Read the model definition and answer for the solid it produces. Units are mm, in the model's axes. Coordinates: 2 decimals unless noted, no trailing zeros. Write each loop counter-clockwise with the first axis right and the second up, starting at its lowest first coordinate (ties: lowest second). Pieces come first, ordered by that corner, then holes.
(1) The part is cut by section B-B, the plane x = 23. Determine the outline of the cut face in (y, z), and give its area (3 significant figures).
(2) The part is cut by section C-C, the plane z = 420. Determine the outline of the cut face in (x, y), and give its area (3 significant figures).
(3) Straight lines are drawn through the part: line 1 along Y through (x, z) = (0, 478.5); line 2 along X through (y, z) = (4, 572.5). For each, find the intervals that lie inside material, in ascending order.
(4) Given pin 1 (1 mm diameter, centred on x = 3, z = 241, fed in from +Y); pin 2 (2 mm diameter, centred on x = -31, y = 34.5, fed in from -Z) (3 decimals); pin 3 (6 mm diameter, centred on y = -1, z = 731, fed in from -X); pin 4 (1 mm diameter, centred on x = 9.5, z = 522.5, fed in from +Y), each flat-ended and moving along its own axis, determine where each tip first touches the part or whether it passes through.
(5) The part is cut by section A-A, the plane y = 31.5. Determine the outline of the cut face in (x, z).
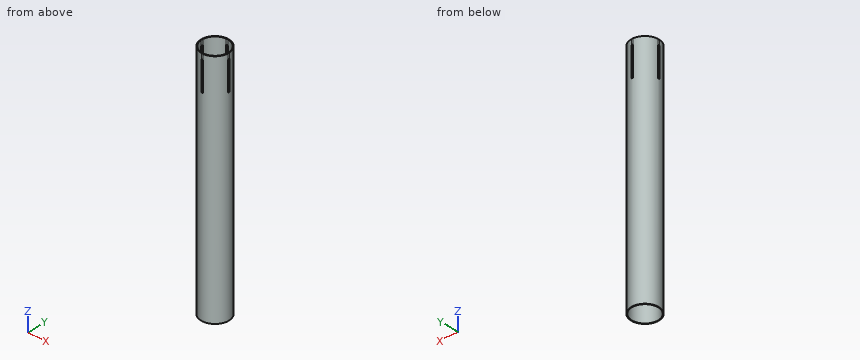
```python
from build123d import *
from build123d.topology import SkipClean

# Parameters (mm, degrees)
SKETCH1_R           = 50.8
SKETCH1_R_2         = 48.26
BOSS_EXTRUDE1_DEPTH = 863.6
CUT_EXTRUDE1_START  = -127
CUT_EXTRUDE1_DEPTH  = 127
BOSS_EXTRUDE2_START = -19.05
BOSS_EXTRUDE2_DEPTH = 19.05


with BuildPart() as part:
    # Sketch1 → Boss-Extrude1 (new body)
    with BuildSketch(Plane.XY):
        Circle(SKETCH1_R)
        Circle(SKETCH1_R_2, mode=Mode.SUBTRACT)
    extrude(amount=BOSS_EXTRUDE1_DEPTH)

    # Sketch2 → Cut-Extrude1 (cut)
    with BuildSketch(Plane.XY.offset(863.6).offset(CUT_EXTRUDE1_START)):
        with BuildLine():
            Line((-3.175, 50.700684167), (-3.175, 48.155445954))
            ThreePointArc((-3.175, 48.155445954), (0, 48.26), (3.175, 48.155445954))
            Line((3.175, 48.155445954), (3.175, 50.700684167))
            ThreePointArc((3.175, 50.700684167), (0, 50.8), (-3.175, 50.700684167))
        make_face()
        with BuildLine():
            Line((-50.700684167, 3.175), (-48.155445954, 3.175))
            ThreePointArc((-48.155445954, 3.175), (-48.26, 0), (-48.155445954, -3.175))
            Line((-48.155445954, -3.175), (-50.700684167, -3.175))
            ThreePointArc((-50.700684167, -3.175), (-50.8, 0), (-50.700684167, 3.175))
        make_face()
        with BuildLine():
            Line((48.155445954, 3.175), (50.700684167, 3.175))
            ThreePointArc((50.700684167, 3.175), (50.8, 0), (50.700684167, -3.175))
            Line((50.700684167, -3.175), (48.155445954, -3.175))
            ThreePointArc((48.155445954, -3.175), (48.26, 0), (48.155445954, 3.175))
        make_face()
        with BuildLine():
            Line((3.175, -48.155445954), (3.175, -50.700684167))
            ThreePointArc((3.175, -50.700684167), (0, -50.8), (-3.175, -50.700684167))
            Line((-3.175, -50.700684167), (-3.175, -48.155445954))
            ThreePointArc((-3.175, -48.155445954), (0, -48.26), (3.175, -48.155445954))
        make_face()
    extrude(amount=CUT_EXTRUDE1_DEPTH, mode=Mode.SUBTRACT)

    # Sketch4 → Boss-Extrude2 (add)
    with SkipClean():  # the faces are left unmerged after this step: merging them gives an invalid solid
        with BuildSketch(Plane.XY.offset(863.6).offset(BOSS_EXTRUDE2_START)):
            with BuildLine():
                Line((-3.175, 50.700684167), (-3.175, 48.155445954))
                ThreePointArc((-3.175, 48.155445954), (0, 48.26), (3.175, 48.155445954))
                Line((3.175, 48.155445954), (3.175, 50.700684167))
                ThreePointArc((3.175, 50.700684167), (0, 50.8), (-3.175, 50.700684167))
            make_face()
            with BuildLine():
                Line((50.700684167, 3.175), (48.155445954, 3.175))
                ThreePointArc((48.155445954, 3.175), (48.26, 0), (48.155445954, -3.175))
                Line((48.155445954, -3.175), (50.700684167, -3.175))
                ThreePointArc((50.700684167, -3.175), (50.8, 0), (50.700684167, 3.175))
            make_face()
            with BuildLine():
                Line((3.175, -50.700684167), (3.175, -48.155445954))
                ThreePointArc((3.175, -48.155445954), (0, -48.26), (-3.175, -48.155445954))
                Line((-3.175, -48.155445954), (-3.175, -50.700684167))
                ThreePointArc((-3.175, -50.700684167), (0, -50.8), (3.175, -50.700684167))
            make_face()
            with BuildLine():
                Line((-48.155445954, 3.175), (-50.700684167, 3.175))
                ThreePointArc((-50.700684167, 3.175), (-50.8, 0), (-50.700684167, -3.175))
                Line((-50.700684167, -3.175), (-48.155445954, -3.175))
                ThreePointArc((-48.155445954, -3.175), (-48.26, 0), (-48.155445954, 3.175))
            make_face()
        extrude(amount=BOSS_EXTRUDE2_DEPTH)


solid = part.part
```
Computed:
1. outline: (-45.3, 0) - (-42.43, 0) - (-42.43, 863.6) - (-45.3, 863.6) - close; (42.43, 0) - (45.3, 0) - (45.3, 863.6) - (42.43, 863.6) - close
1. area: 4,950 mm2
2. outline: circle Ø101.6 at (0, 0); hole circle Ø96.52 at (0, 0)
2. area: 790 mm2
3. line 1: y = -50.8 to -48.26, 48.26 to 50.8
3. line 2: x = -50.64 to -48.09, 48.09 to 50.64
4. pin 1: stops at y = 50.74
4. pin 2: passes through
4. pin 3: stops at x = -50.8
4. pin 4: stops at y = 50
5. outline: (-39.85, 0) - (-36.56, 0) - (-36.56, 863.6) - (-39.85, 863.6) - close; (36.56, 0) - (39.85, 0) - (39.85, 863.6) - (36.56, 863.6) - close
